from build123d import *

# Parameters (mm, degrees)
BOX009_W               = 2
BOX009_H               = 6
BOX009_DEPTH           = 19
BOX009_PLACEMENT_ANGLE = 25
BOX005_W               = 8
BOX005_H               = 9
BOX005_DEPTH           = 20
BOX007_W               = 125
BOX007_H               = 8
BOX007_DEPTH           = 60
BOX007_PLACEMENT_ANGLE = 25
BOX008_W               = 129
BOX008_H               = 47
BOX008_DEPTH           = 10
BOX004_W               = 8
BOX004_H               = 9
BOX004_DEPTH           = 20
BOX006_W               = 120
BOX006_H               = 20
BOX006_DEPTH           = 46
BOX003_W               = 129
BOX003_H               = 20
BOX003_DEPTH           = 67
BOX003_PLACEMENT_ANGLE = 25


with BuildPart() as cube009:
    # Box009 → Box009 (new body)
    with BuildSketch(Plane.XY):
        with Locations((1, 3)):
            Rectangle(BOX009_W, BOX009_H)
    extrude(amount=BOX009_DEPTH)


with BuildPart() as cube009_1:
    # Box009 placement: moved
    add(cube009.part.moved(Location((-9, -15, 92))).rotate(Axis((-9, -15, 92), (-1, 0, 0)), BOX009_PLACEMENT_ANGLE))


with BuildPart() as cube005:
    # Box005 → Box005 (new body)
    with BuildSketch(Plane(origin=(103, 8, 70), x_dir=(1, 0, 0), z_dir=(0, 0, 1))):
        with Locations((4, 4.5)):
            Rectangle(BOX005_W, BOX005_H)
    extrude(amount=BOX005_DEPTH)


with BuildPart() as cube007:
    # Box007 → Box007 (new body)
    with BuildSketch(Plane.XY):
        with Locations((62.5, 4)):
            Rectangle(BOX007_W, BOX007_H)
    extrude(amount=BOX007_DEPTH)


with BuildPart() as cube007_1:
    # Box007 placement: moved
    add(cube007.part.moved(Location((-7, -24, 74))).rotate(Axis((-7, -24, 74), (-1, 0, 0)), BOX007_PLACEMENT_ANGLE))


with BuildPart() as cube008:
    # Box008 → Box008 (new body)
    with BuildSketch(Plane(origin=(-9, -27, 60), x_dir=(1, 0, 0), z_dir=(0, 0, 1))):
        with Locations((64.5, 23.5)):
            Rectangle(BOX008_W, BOX008_H)
    extrude(amount=BOX008_DEPTH)


with BuildPart() as fusion004:
    # Box004 → Box004 (new body)
    with BuildSketch(Plane(origin=(-1, 8, 70), x_dir=(1, 0, 0), z_dir=(0, 0, 1))):
        with Locations((4, 4.5)):
            Rectangle(BOX004_W, BOX004_H)
    extrude(amount=BOX004_DEPTH)

    # Fusion004: union Cube005, Cube007, Cube008
    add(cube005.part)
    add(cube007_1.part)
    add(cube008.part)


with BuildPart() as cube006:
    # Box006 → Box006 (new body)
    with BuildSketch(Plane(origin=(-5, 0, 70), x_dir=(1, 0, 0), z_dir=(0, 0, 1))):
        with Locations((60, 10)):
            Rectangle(BOX006_W, BOX006_H)
    extrude(amount=BOX006_DEPTH)


with BuildPart() as iphonehalterung:
    # Box003 → Box003 (new body)
    with BuildSketch(Plane.XY):
        with Locations((64.5, 10)):
            Rectangle(BOX003_W, BOX003_H)
    extrude(amount=BOX003_DEPTH)


with BuildPart() as iphonehalterung_1:
    # Box003 placement: moved
    add(iphonehalterung.part.moved(Location((-9, -25, 70))).rotate(Axis((-9, -25, 70), (-1, 0, 0)), BOX003_PLACEMENT_ANGLE))

    # Fusion003: union Cube006
    add(cube006.part)

    # Cut001: cut Fusion004
    add(fusion004.part, mode=Mode.SUBTRACT)

    # Cut002: cut Cube009
    add(cube009_1.part, mode=Mode.SUBTRACT)


solid = iphonehalterung_1.part
CAD build for the part. Positions are in the model's coordinates, mm. A direction names the side the tool comes from. Coordinates: 2 decimals unless noted, no trailing zeros. Order: outer loops, then holes, each group sorted by start corner. A loop starts at its lowest first (then second) coordinate and runs counter-clockwise, first axis right, second up.
Item 1: Two-plate mould, pull along X, no slides. Class faces 1 (the face through (107, 17, 80)), 2 (the face through (120, -2, 96)), 3 (the face through (54.597, 12.505, 126.437)): +X half, -X half, draft (parallel to the pull), parting line (faces both ways), or undercut.
Check sheet entries:
face 1: undercut
face 2: +X half
face 3: draft
Item 2: Drill centre lines: L1, parallel to Y at x = -0.5, z = 73.5; L2, parallel to X at y = 13, z = 101; L3, parallel to Z at x = 97, y = 6.5. Where is each one in solid material? Low to high.
Check sheet entries:
L1: y = -23.37 to -22.93, -15.41 to -1.3, 0 to 8, 17 to 20
L2: x = -5 to 115
L3: z = 70 to 120.48, 125.98 to 129.24
Item 3: Band-saw the part on D-D on y = -8. List the corners of the cut face in (x, z).
Check sheet entries:
outline: (-9, 70) - (120, 70) - (120, 106.46) - (118, 106.46) - (118, 89.38) - (-7, 89.38) - (-7, 92.81) - (-9, 92.81) - close
Item 4: Band-saw the part on C-C on z = 94.5. List the corners of the cut face in (x, y).
Check sheet entries:
outline: (-9, -7.21) - (-7, -7.21) - (-7, -5.61) - (118, -5.61) - (118, -13.58) - (120, -13.58) - (120, 8.49) - (115, 8.49) - (115, 20) - (-5, 20) - (-5, 8.49) - (-9, 8.49) - close
Item 5: 3-axis set-ups, long thin cutter, end or side, ignore diameter. For faces 4 (the face through (-8.014, -12.138, 90.666)), 5 (the face through (-5, 12, 88)), 6 (the face through (115, 12, 88)), 7 (the face through (3, 8, 80)): which of +Z, -Z, +X, -X, +Y, -Y reach the whole face in a straight line?
Check sheet entries:
face 4: +Z, -X
face 5: -Z, -X, +Y
face 6: -Z, +X, +Y
face 7: -Z
Item 6: Pin check, flat tips, straight feed: pin 1 Ø12 at (x, z) = (103, 79.5) entering from +Y; pin 2 Ø10 at (x, y) = (48.5, 2.5) entering from +Z; pin 3 Ø6 at (x, z) = (106.5, 99.5) entering from -Y. Stop position of each tip, or through.
Check sheet entries:
pin 1: stops at y = 20
pin 2: stops at z = 130.72
pin 3: stops at y = -4.68
Item 7: Band-saw the part on B-B on y = 5.5. List the corners of the cut face in (x, z).
Check sheet entries:
outline: (-9, 88.08) - (-5, 88.08) - (-5, 70) - (115, 70) - (115, 88.08) - (120, 88.08) - (120, 129.7) - (-9, 129.7) - close; hole (-7, 118.33) - (118, 118.33) - (118, 126.45) - (-7, 126.45) - close
Item 8: Band-saw the part on A-A on x = 84.5. List the corners of the cut face in (y, z).
Check sheet entries:
outline: (-25, 70) - (-2.93, 70) - (0, 76.29) - (0, 70) - (20, 70) - (20, 116) - (18.52, 116) - (21.44, 122.27) - (3.32, 130.72) - (2.07, 128.05) - (8.61, 125) - (-16.75, 70.62) - (-23.29, 73.67) - close
